```python
from build123d import *

# Parameters (mm, degrees)
SKICA1_W                     = 37.3
SKICA1_H                     = 15.8
P_IDAT_VYSUNUT_M1_DEPTH      = 1.5
SKICA1_3_W                   = 27.2
SKICA1_3_H                   = 13.1
P_IDAT_VYSUNUT_M2_DEPTH      = 1
SKICA2_W                     = 2.56
SKICA2_H                     = 10.24
P_IDAT_VYSUNUT_M3_DEPTH      = 2.7
P_IDAT_VYSUNUT_M4_DEPTH      = 1.8
P_IDAT_VYSUNUT_M4_DEPTH_BACK = 5.8
SKICA3_W                     = 0.65
SKICA3_H                     = 0.65
SKICA4_W                     = 0.65
SKICA4_H                     = 0.65
P_IDAT_VYSUNUT_M5_DEPTH      = 6.7
ZAOBLIT1_R                   = 1
ZAOBLIT2_R                   = 0.5
P_IDAT_VYSUNUT_M6_DEPTH      = 0.6
P_IDAT_VYSUNUT_M6_DEPTH_BACK = 3.8
SKICA5_W                     = 29.4
SKICA5_H                     = 16.4
SKICA6_W                     = 6.3
SKICA6_H                     = 16.4
ODEBRAT_VYSUNUT_M1_DEPTH     = 0.9
ZAOBLIT3_R                   = 5
ZAOBLIT4_R                   = 5
SKICA7_W                     = 4
SKICA7_H                     = 16.4
ODEBRAT_VYSUNUT_M2_DEPTH     = 0.9
ZAOBLIT7_R                   = 5
ZAOBLIT8_R                   = 5
ZAOBLIT5_R                   = 2.5
ZAOBLIT6_R                   = 0.6
ZAOBLIT9_R                   = 0.5
ZAOBLIT10_R                  = 0.5


with BuildPart() as part:
    # Skica1 → Přidat vysunutím1 (new body)
    with BuildSketch(Plane.XY):
        Rectangle(SKICA1_W, SKICA1_H)
    extrude(amount=-P_IDAT_VYSUNUT_M1_DEPTH)

    # Skica1<3> → Přidat vysunutím2 (add)
    with BuildSketch(Plane.XY):
        with Locations((-5.05, 0)):
            Rectangle(SKICA1_3_W, SKICA1_3_H)
    extrude(amount=P_IDAT_VYSUNUT_M2_DEPTH)

    # Skica2 → Přidat vysunutím3 (add)
    with BuildSketch(Plane.XY):
        with Locations((17.37, 0)):
            Rectangle(SKICA2_W, SKICA2_H)
    extrude(amount=P_IDAT_VYSUNUT_M3_DEPTH)

    # Skica3 → Přidat vysunutím4 (add, two sides: drawn at the far end of the back side and taken through both)
    with BuildSketch(Plane.XY.offset(2.7).offset(-P_IDAT_VYSUNUT_M4_DEPTH_BACK)):
        with Locations((17.37, -3.84)):
            Rectangle(SKICA3_W, SKICA3_H)
        with Locations((17.37, -1.28)):
            Rectangle(SKICA3_W, SKICA3_H)
        with Locations((17.37, 1.28)):
            Rectangle(SKICA3_W, SKICA3_H)
        with Locations((17.37, 3.84)):
            Rectangle(SKICA3_W, SKICA3_H)
    extrude(amount=P_IDAT_VYSUNUT_M4_DEPTH + P_IDAT_VYSUNUT_M4_DEPTH_BACK)

    # Skica4 → Přidat vysunutím5 (add)
    with BuildSketch(Plane(origin=(17.695, 0, 0), x_dir=(0, 0, -1), z_dir=(1, 0, 0))):
        with Locations((-4.175, -3.84)):
            Rectangle(SKICA4_W, SKICA4_H)
        with Locations((-4.175, -1.28)):
            Rectangle(SKICA4_W, SKICA4_H)
        with Locations((-4.175, 1.28)):
            Rectangle(SKICA4_W, SKICA4_H)
        with Locations((-4.175, 3.84)):
            Rectangle(SKICA4_W, SKICA4_H)
    extrude(amount=P_IDAT_VYSUNUT_M5_DEPTH)

    # Zaoblit1
    zaoblit1_edges = [part.edges().sort_by_distance(p)[0] for p in [
        (17.045, 3.84, 4.5),
        (17.045, -3.84, 4.5),
        (17.045, -1.28, 4.5),
        (17.045, 1.28, 4.5),
    ]]
    fillet(zaoblit1_edges, radius=ZAOBLIT1_R)

    # Zaoblit2
    zaoblit2_edges = [part.edges().sort_by_distance(p)[0] for p in [
        (17.695, -3.84, 3.85),
        (17.695, -1.28, 3.85),
        (17.695, 1.28, 3.85),
        (17.695, 3.84, 3.85),
    ]]
    fillet(zaoblit2_edges, radius=ZAOBLIT2_R)

    # Skica5 → Přidat vysunutím6 (add, two sides: drawn at the far end of the back side and taken through both)
    with BuildSketch(Plane(origin=(0, 0, -1.5), x_dir=(-1, 0, 0), z_dir=(0, 0, -1)).offset(-P_IDAT_VYSUNUT_M6_DEPTH_BACK)):
        with Locations((-0.95, 0)):
            Rectangle(SKICA5_W, SKICA5_H)
    extrude(amount=P_IDAT_VYSUNUT_M6_DEPTH + P_IDAT_VYSUNUT_M6_DEPTH_BACK)

    # Skica6 → Odebrat vysunutím1 (cut)
    with BuildSketch(Plane.XY.offset(2.3)):
        with Locations((12.5, 0)):
            Rectangle(SKICA6_W, SKICA6_H)
    extrude(amount=-ODEBRAT_VYSUNUT_M1_DEPTH, mode=Mode.SUBTRACT)

    # Zaoblit3
    # the kernel refuses this fillet: 5 mm, written as the material it adds along each edge
    with BuildSketch(Plane(origin=(9.35, -8.2, 1.4), x_dir=(1, 0, 0), z_dir=(0, 1, 0))) as zaoblit3_piece_1:
        with BuildLine():
            CenterArc((2.861817604, -5), ZAOBLIT3_R, 90, 34.915206247)
            Line((0, -0.9), (-0.057236352, -0.818))
            ThreePointArc((-0.057236352, -0.818), (-0.1, -0.45), (-0.1, 0))
            Line((-0.1, 0), (0, 0.1))
            Line((0, 0.1), (2.861817604, 0.1))
            Line((2.861817604, 0.1), (2.861817604, 0))
        make_face()
    extrude(amount=16.4)

    # Zaoblit4
    zaoblit4_edges = [part.edges().sort_by_distance(p)[0] for p in [
        (9.35, 0, 2.3),
    ]]
    fillet(zaoblit4_edges, radius=ZAOBLIT4_R)

    # Skica7 → Odebrat vysunutím2 (cut)
    with BuildSketch(Plane.XY.offset(2.3)):
        with Locations((-11.75, 0)):
            Rectangle(SKICA7_W, SKICA7_H)
    extrude(amount=-ODEBRAT_VYSUNUT_M2_DEPTH, mode=Mode.SUBTRACT)

    # Zaoblit7
    # the kernel refuses this fillet: 5 mm, written as the material it adds along each edge
    with BuildSketch(Plane(origin=(-9.75, 8.2, 1.4), x_dir=(-1, 0, 0), z_dir=(0, -1, 0))) as zaoblit7_piece_1:
        with BuildLine():
            CenterArc((2.861817604, -5), ZAOBLIT7_R, 90, 34.915206247)
            Line((0, -0.9), (0, 0))
            Line((0, 0), (2.861817604, 0))
        make_face()
    extrude(amount=16.4)

    # Zaoblit8
    zaoblit8_edges = [part.edges().sort_by_distance(p)[0] for p in [
        (-9.75, 0, 2.3),
    ]]
    fillet(zaoblit8_edges, radius=ZAOBLIT8_R)

    # Zaoblit5
    zaoblit5_edges = [part.edges().sort_by_distance(p)[0] for p in [
        (13.930908802, 8.2, 1.4),
        (13.930908802, -8.2, 1.4),
        (11.151157432, -8.2, 1.513794929),
        (11.151157432, 8.2, 1.513794929),
        (-0.2, -8.2, 2.3),
        (9.126395288, -8.2, 2.186205071),
        (9.126395288, 8.2, 2.186205071),
        (-13.180908802, -8.2, 1.4),
        (-13.180908802, 8.2, 1.4),
        (-11.551157432, 8.2, 1.513794929),
        (-11.551157432, -8.2, 1.513794929),
        (-0.2, 8.2, 2.3),
        (-9.526395288, 8.2, 2.186205071),
        (-9.526395288, -8.2, 2.186205071),
    ]]
    fillet(zaoblit5_edges, radius=ZAOBLIT5_R)

    # Zaoblit6
    zaoblit6_edges = [part.edges().sort_by_distance(p)[0] for p in [
        (0.95, 8.2, -2.1),
        (0.95, -8.2, -2.1),
    ]]
    fillet(zaoblit6_edges, radius=ZAOBLIT6_R)

    # Zaoblit9
    zaoblit9_edges = [part.edges().sort_by_distance(p)[0] for p in [
        (18.65, -5.12, 1.35),
        (18.65, 5.12, 1.35),
        (16.09, 5.12, 1.35),
        (16.09, -5.12, 1.35),
    ]]
    fillet(zaoblit9_edges, radius=ZAOBLIT9_R)

    # Zaoblit10
    zaoblit10_edges = [part.edges().sort_by_distance(p)[0] for p in [
        (17.695, 3.84, -1.5),
        (17.37, 3.515, -1.5),
        (17.045, 3.84, -1.5),
        (17.37, 4.165, -1.5),
        (17.045, -3.84, -1.5),
        (17.37, -3.515, -1.5),
        (17.695, -3.84, -1.5),
        (17.37, -4.165, -1.5),
        (17.045, -1.28, -1.5),
        (17.37, -0.955, -1.5),
        (17.695, -1.28, -1.5),
        (17.37, -1.605, -1.5),
        (17.695, 1.28, -1.5),
        (17.37, 0.955, -1.5),
        (17.045, 1.28, -1.5),
        (17.37, 1.605, -1.5),
    ]]
    fillet(zaoblit10_edges, radius=ZAOBLIT10_R)


solid = part.part
```
Input: part model. Units: mm. Frame: model coordinates. A direction names the side the tool comes from. Give positions to 0.01 mm unless a question says otherwise; leave off trailing zeros. Write each loop counter-clockwise with the first axis right and the second up, starting at its lowest first coordinate (ties: lowest second). Pieces come first, ordered by that corner, then holes. Notation, with made-up numbers: (17.5, 30.5) - (63.5, 30.5) arc R20 cw to (63.5, 43.5) - close; hole circle Ø8 at (25.25, -34). An arc over 180 degrees is marked (long way). Write item = value, one per line. Start each with the question number.
1) Cut plane B-B (x = 14.5). Return loops of the section in (y, z), and give its area (3 significant figures).
2) Material intervals for L1, parallel to X at y = -4.5, z = 2.5; L2, parallel to X at y = -1.25, z = 3.25 (3 decimals); L3, parallel to Z at x = -1, y = 5.5, sorted ascending. Write a range as [from, to].
3) Reachability of faces 4 (the face through (17, 7.9, -1)), 5 (the face through (-16, -7, 0)), 6 (the face through (17, 5.12, 1)), 7 (the face through (20, 1.605, 4)), 8 (the face through (0, 0, 2.3)) from +Z, -Z, +X, -X, +Y, -Y: full face, straight path, thin tool, end or side. Return the list, or none.
4) Cut plane C-C (y = 0). Return loops of the section in (x, z), and give its area (3 significant figures).
5) Draft query along Y for faces 1 (the face through (-16.2, 6.55, 0.5)), 2 (the face through (-13.173, -7.487, 0.648)), 3 (the face through (20, -3.515, 4)). Return one class per face: pulls with the +Y half, pulls with the -Y half, needs draft (parallel to the pull), parting line crosses it, or undercut.
6) Cut plane A-A (z = -2.5). Return loops of the section in (x, y) (3 decimals), and give its area (3 significant figures).
7) Cut plane D-D (x = -3). Return loops of the section in (y, z).
8) Pin query (flat end, axial travel): pin 1 (0.8 mm diameter, centred on x = -15, z = -0.5, fed in from -Y); pin 2 (6 mm diameter, centred on x = 1.5, y = 1.5, fed in from +Z); pin 3 (0.5 mm diameter, centred on x = 17.5, z = 2, fed in from -Y). Return the tip coordinate at first contact, or that it passes through.
Answers follow:
q1.outline = (-8.2, -1.5) arc R0.6 ccw to (-7.6, -2.1) - (7.6, -2.1) arc R0.6 ccw to (8.2, -1.5) - (8.2, -1.1) arc R2.5 ccw to (5.7, 1.4) - (-5.7, 1.4) arc R2.5 ccw to (-8.2, -1.1) - close
q1.area = 54.6 mm^2
q2.L1 = [16.09, 18.65]
q2.L2 = [17.045, 17.695]
q2.L3 = [-2.1, 2.3]
q3.face_4 = +Z, -Z, +X, +Y
q3.face_5 = +Z, -X, -Y
q3.face_6 = +Z, +X, +Y
q3.face_7 = +Z, +X, -X
q3.face_8 = +Z, -X, +Y, -Y
q4.outline = (-18.65, -1.5) - (-13.75, -1.5) - (-13.75, -2.1) - (15.65, -2.1) - (15.65, -1.5) - (18.65, -1.5) - (18.65, 2.7) - (16.09, 2.7) - (16.09, 0) - (15.65, 0) - (15.65, 1.4) - (12.21, 1.4) arc R5 cw to (10.14, 1.85) arc R5 ccw to (8.07, 2.3) - (-8.47, 2.3) arc R5 ccw to (-10.54, 1.85) arc R5 cw to (-12.61, 1.4) - (-13.75, 1.4) - (-13.75, 1) - (-18.65, 1) - close
q4.area = 145 mm^2
q5.face_1 = pulls with the +Y half
q5.face_2 = pulls with the -Y half
q5.face_3 = undercut
q6.outline = (17.045, -4.165) - (17.695, -4.165) - (17.695, -3.515) - (17.045, -3.515) - close; (17.045, -1.605) - (17.695, -1.605) - (17.695, -0.955) - (17.045, -0.955) - close; (17.045, 0.955) - (17.695, 0.955) - (17.695, 1.605) - (17.045, 1.605) - close; (17.045, 3.515) - (17.695, 3.515) - (17.695, 4.165) - (17.045, 4.165) - close
q6.area = 1.69 mm^2
q7.outline = (-8.2, -1.5) arc R0.6 ccw to (-7.6, -2.1) - (7.6, -2.1) arc R0.6 ccw to (8.2, -1.5) - (8.2, -0.2) arc R2.5 ccw to (5.7, 2.3) - (-5.7, 2.3) arc R2.5 ccw to (-8.2, -0.2) - close
q8.pin_1 = -7.9
q8.pin_2 = 2.3
q8.pin_3 = -5.12
